Part model, mm, in its own coordinate system. A direction names the side the tool comes from. Give positions to 0.01 mm unless a question says otherwise; leave off trailing zeros. Order: outer loops, then holes, each group sorted by start corner. A loop starts at its lowest first (then second) coordinate and runs counter-clockwise, first axis right, second up.
1. Drop flat-ended pins along their axis: pin 1 Ø1 at (x, y) = (-12.5, -23.5) entering from -Z; pin 2 Ø4 at (y, z) = (-16.5, 21) entering from -X; pin 3 Ø9 at (x, y) = (0, -16.06) entering from -Z; pin 4 Ø8 at (x, z) = (13, 21) entering from -Y. Give the stop position or say it passes through.
2. Probe line 1 (Z direction, x = 6, y = -29.5); line 2 (Y direction, x = 0, z = 3.05); line 3 (Y direction, x = 0, z = 13.5). List the from-to ranges inside material, lowest first.
3. Slice it at B-B on z = 2.5. List the corners of the cut face in (x, y) (3 decimals).
4. Slice it at A-A on z = 23.5. List the corners of the cut face in (x, y), and give its area (3 significant figures).
5. Mould opens along X. For faces 1 (the cylindrical face through (-4.13, -35.017, 22.935)), 2 (the cylindrical face through (-8.259, -41.387, 10.499)), 3 (the flat face through (-24, 7, 27.9)) say: +X half, -X half, draft (parallel to the pull), parting line (faces both ways), or undercut.
6. Which spindle directions (+Z, -Z, +X, -X, +Y, -Y) get a long thin tool onto all of the face, cutting with end or side? Do faces 4 (the cylindrical face through (-30.92, 7.6, 26.63)), 5 (the flat face through (22, 8, 27.9)), 6 (the cylindrical face through (-0.744, -21.722, 1.923)). Say none if no direction does.
from build123d import *

# Parameters (mm, degrees)
F0_R      = 38.1
F2_DEPTH  = 25.4
F3_R      = 4.104163056
F4_R      = 7.676399804
F4_R_2    = 7.4730209118
F4_R_3    = 7.9111301116
F4_R_4    = 7.0349890874
F6_DEPTH  = 2.5
F7_R      = 19.05
F8_DEPTH  = 5
F9_R      = 5.715
F10_DEPTH = 3.9
F11_R     = 2.9751470693
F12_DEPTH = 24.001


# Not quite as in the source:
# - a feature names something its author has since deleted; it is built from what else it names


with BuildPart() as f2:
    # F0 (on Top) → F2 (new body)
    with BuildSketch(Plane.XY):
        with Locations((0, -4.1931332196)):
            Circle(F0_R)
    extrude(amount=F2_DEPTH)

    # F3
    f3_edges = [f2.edges().sort_by_distance(p)[0] for p in [
        (-38.1, -4.193133, 25.4),
    ]]
    fillet(f3_edges, radius=F3_R)

    # F4 (on face) → F6 (join)
    with BuildSketch(Plane.XY.offset(25.4)):
        with Locations((-9.9296038883, 16.6010573738)):
            Circle(F4_R)
        with Locations((6.8266042386, 15.9804562879)):
            Circle(F4_R_2)
        with Locations((22.3416063405, 8.2229533103)):
            Circle(F4_R_3)
        with Locations((-23.8931100186, 7.2920526448)):
            Circle(F4_R_4)
    extrude(amount=F6_DEPTH)

    # F7 (on face) → F8 (cut)
    with BuildSketch(Plane.XY.offset(25.4)):
        with Locations((0, -16.4202762372)):
            Circle(F7_R)
    extrude(amount=-F8_DEPTH, mode=Mode.SUBTRACT)

    # F9 (on face) → F10 (cut)
    with BuildSketch(Plane(origin=(0, 0, 0), x_dir=(1, 0, 0), z_dir=(0, 0, -1))):
        with Locations((0, 16.0560380752)):
            Circle(F9_R)
    extrude(amount=-F10_DEPTH, mode=Mode.SUBTRACT)

    # F11 (on face) → F12 (cut, through all)
    with BuildSketch(Plane(origin=(0, 0, 3.9), x_dir=(1, 0, 0), z_dir=(0, 0, -1))):
        with Locations((0, 16.0560380752)):
            Circle(F11_R)
    extrude(amount=-F12_DEPTH, mode=Mode.SUBTRACT)


solid = f2.part
Data:
1. pin 1: stops at z = 0
1. pin 2: stops at x = -36.68
1. pin 3: stops at z = 3.9
1. pin 4: stops at y = -41.21
2. line 1: z = 0 to 20.4
2. line 2: y = -42.29 to -21.77, -10.34 to 33.91
2. line 3: y = -42.29 to -19.03, -13.08 to 33.91
3. outline: circle Ø76.2 at (0, -4.193); hole circle Ø11.43 at (0, -16.056)
4. outline: circle Ø74.92 at (0, -4.19); hole circle Ø38.1 at (0, -16.42)
4. area: 3,270 mm2
5. face 1: undercut
5. face 2: parting line
5. face 3: draft
6. face 4: +Z
6. face 5: +Z, +X, -X, +Y, -Y
6. face 6: -Z
